```python
from build123d import *

# Parameters (mm, degrees)
F0_W     = 50
F0_H     = 25
F0_W_2   = 90
F0_H_2   = 45
F1_DEPTH = 4
F2_DEPTH = 2
F5_DEPTH = 2.001
F7_R     = 5
F0_R     = 1.6666666667
F8_DEPTH = 4
F9_DEPTH = 2


# Not quite as in the source:
# - a feature names something its author has since deleted; it is built from what else it names


with BuildPart() as f1:
    # F0 (on Top) → F1 (new body)
    with BuildSketch(Plane.XY):
        Polygon((-53, -84.5), (53, -84.5), (53, -2.5), (5, -2.5), (-5, -2.5), (-53, -2.5), align=None)
        with Locations((0, -68)):
            Rectangle(F0_W, F0_H, mode=Mode.SUBTRACT)
        with Locations((0, -29)):
            Rectangle(F0_W_2, F0_H_2, mode=Mode.SUBTRACT)
    extrude(amount=F1_DEPTH)

    # F0 (on Top) → F2 (join)
    with BuildSketch(Plane.XY):
        with Locations((0, -68)):
            Rectangle(F0_W, F0_H)
        with Locations((0, -29)):
            Rectangle(F0_W_2, F0_H_2)
    extrude(amount=F2_DEPTH)

    # F4 (on offset) → F5 (cut, through all)
    with BuildSketch(Plane.XY.offset(2)):
        with BuildLine():
            Line((-4.1848091993, 17.7334633669), (-4.1848091993, 13.1759698881))
            ThreePointArc((-4.1848091993, 13.1759698881), (-0.249754072, 9.1237647174), (5, 11.2082569299))
            Line((5, 11.2082569299), (5, 17.5))
            ThreePointArc((5, 17.5), (3.3860967443, 17.9195789218), (1.7383729014, 18.1759698881))
            Line((1.7383729014, 18.1759698881), (-1.7383729014, 18.1759698881))
            ThreePointArc((-1.7383729014, 18.1759698881), (-2.9698441971, 18.0003448764), (-4.1848091993, 17.7334633669))
        make_face()
        with BuildLine():
            ThreePointArc((5, 11.2082569299), (-0.249754072, 9.1237647174), (-4.1848091993, 13.1759698881))
            Line((-4.1848091993, 13.1759698881), (-4.1848091993, 17.7334633669))
            ThreePointArc((-4.1848091993, 17.7334633669), (-12.2142757372, 12.9486427976), (-16.4107558429, 4.5966133744))
            Line((-16.4107558429, 4.5966133744), (-5, -2.5))
            Line((-5, -2.5), (5, -2.5))
            Line((5, -2.5), (5, 11.2082569299))
        make_face()
    extrude(amount=-F5_DEPTH, mode=Mode.SUBTRACT)

    # F7
    f7_edges = [f1.edges().sort_by_distance(p)[0] for p in [
        (53, -84.5, 2),
        (-53, -84.5, 2),
        (-53, -2.5, 2),
        (53, -2.5, 2),
    ]]
    fillet(f7_edges, radius=F7_R)

    # F0 (on Top) → F8 (join)
    with BuildSketch(Plane.XY):
        with BuildLine():
            Line((-5, -2.5), (5, -2.5))
            Line((5, -2.5), (5, 17.5))
            ThreePointArc((5, 17.5), (0, 22.5), (-5, 17.5))
            Line((-5, 17.5), (-5, -2.5))
        make_face()
        with Locations((0, 17.5)):
            Circle(F0_R, mode=Mode.SUBTRACT)
    extrude(amount=F8_DEPTH)

    # F0 (on Top) → F9 (cut)
    with BuildSketch(Plane.XY):
        with BuildLine():
            Line((-5, -2.5), (5, -2.5))
            Line((5, -2.5), (5, 17.5))
            ThreePointArc((5, 17.5), (0, 22.5), (-5, 17.5))
            Line((-5, 17.5), (-5, -2.5))
        make_face()
        with Locations((0, 17.5)):
            Circle(F0_R, mode=Mode.SUBTRACT)
    extrude(amount=F9_DEPTH, mode=Mode.SUBTRACT)


solid = f1.part
```
The model under review builds one solid part; all positions refer to its coordinate system, in mm. A direction names the side the tool comes from. Give positions to 0.01 mm unless a question says otherwise; leave off trailing zeros. Write each loop counter-clockwise with the first axis right and the second up, starting at its lowest first coordinate (ties: lowest second). Pieces come first, ordered by that corner, then holes.
(1) Tool access review of faces 5 (the flat face through (-1, -29, 2)), 6 (the flat face through (53, -44, 2)), 7 (the flat face through (0, 10, 2)): name each direction out of +Z, -Z, +X, -X, +Y, -Y from which nothing blocks a thin tool from reaching the whole face with its end or side.
(2) To check wall thickness, follow L1, parallel to Y at x = -14, z = 3; L2, parallel to Y at x = 0, z = 2.75; L3, parallel to Y at x = 29, z = 2.55. State the ranges of each line that lie inside material, in increasing order.
(3) The part is to be moulded in two halves that separate along X. For faces 1 (the cylindrical face through (-0.217, 19.152, 2.986)), 2 (the cylindrical face through (0.1, 22.5, 3)), 3 (the flat face through (-1, -54, 4)), 4 (the flat face through (0, -68, 2)), say which applies: released by +X, released by -X, zero draft, split by the parting line, or undercut.
(4) For P1, Ø2, axis at x = 1, z = 2.5, coming from the +Y side; P2, Ø1, axis at y = 7.5, z = 3, coming from the -X side; P3, Ø5, axis at x = 2, y = 15, coming from the -Z side; P4, Ø2, axis at x = 10, z = 3.5, coming from the +Y side, all flat-tipped, find the tip position at first contact; note any pin that passes through.
(5) Consider section A-A, the plane z = 2.85. Give the boundary of the cut face in (x, y), and give its area (3 significant figures).
(6) Consider section B-B, the plane x = 0. Give the boundary of the cut face in (y, z).
(7) Consider section D-D, the plane x = -27.5. Give the boundary of the cut face in (y, z), and give its area (3 significant figures).
(8) Consider section C-C, the plane y = -17. Give the boundary of the cut face in (x, z), and give its area (3 significant figures).
Returned:
1. face 5: +Z
1. face 6: +Z, -Z, +X, +Y, -Y
1. face 7: -Z, +X, -X, +Y
2. L1: y = -84.5 to -80.5, -55.5 to -51.5, -6.5 to -2.5
2. L2: y = -84.5 to -80.5, -55.5 to -51.5, -6.5 to 15.83, 19.17 to 22.5
2. L3: y = -84.5 to -51.5, -6.5 to -2.5
3. face 1: undercut
3. face 2: split by the parting line
3. face 3: zero draft
3. face 4: undercut
4. P1: stops at y = 22.5
4. P2: stops at x = -5
4. P3: stops at z = 2
4. P4: stops at y = -2.5
5. outline: (-53, -79.5) arc R5 ccw to (-48, -84.5) - (48, -84.5) arc R5 ccw to (53, -79.5) - (53, -7.5) arc R5 ccw to (48, -2.5) - (5, -2.5) - (5, 17.5) arc R5 ccw to (-5, 17.5) - (-5, -2.5) - (-48, -2.5) arc R5 ccw to (-53, -7.5) - close; hole (-45, -51.5) - (45, -51.5) - (45, -6.5) - (-45, -6.5) - close; hole (-25, -80.5) - (25, -80.5) - (25, -55.5) - (-25, -55.5) - close; hole circle Ø3.33 at (0, 17.5)
5. area: 3,600 mm2
6. outline: (-84.5, 0) - (-2.5, 0) - (-2.5, 2) - (15.83, 2) - (15.83, 4) - (-6.5, 4) - (-6.5, 2) - (-51.5, 2) - (-51.5, 4) - (-55.5, 4) - (-55.5, 2) - (-80.5, 2) - (-80.5, 4) - (-84.5, 4) - close; (19.17, 2) - (22.5, 2) - (22.5, 4) - (19.17, 4) - close
7. outline: (-84.5, 0) - (-2.5, 0) - (-2.5, 4) - (-6.5, 4) - (-6.5, 2) - (-51.5, 2) - (-51.5, 4) - (-84.5, 4) - close
7. area: 238 mm2
8. outline: (-53, 0) - (53, 0) - (53, 4) - (45, 4) - (45, 2) - (-45, 2) - (-45, 4) - (-53, 4) - close
8. area: 244 mm2
